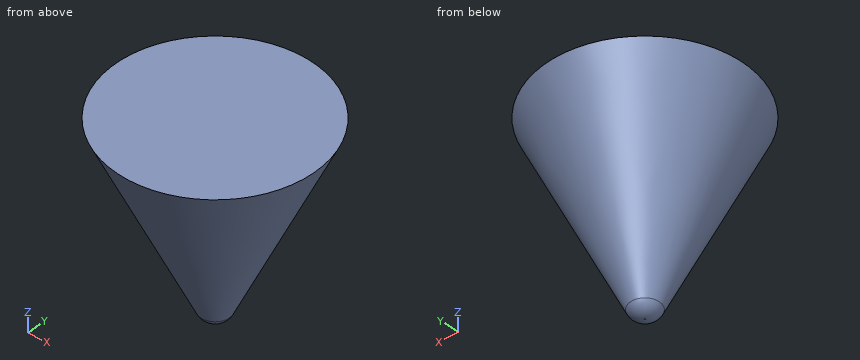
from build123d import *

# Parameters (mm, degrees)
F1_R     = 4.699
F2_DEPTH = 6.35
F2_TAPER = 25
F3_R     = 2.54
F4_R     = 4.699
F5_DEPTH = 25.4
F5_TAPER = -25


with BuildPart() as f2:
    # F1 (on offset) → F2 (new body)
    with BuildSketch(Plane.XY.offset(-25.4)):
        Circle(F1_R)
    extrude(amount=-F2_DEPTH, taper=F2_TAPER)

    # F3
    f3_edges = [f2.edges().sort_by_distance(p)[0] for p in [
        (-1.737946, 0, -31.75),
    ]]
    fillet(f3_edges, radius=F3_R)

    # F4 (on offset) → F5 (join)
    with BuildSketch(Plane.XY.offset(-25.4)):
        Circle(F4_R)
    extrude(amount=F5_DEPTH, taper=F5_TAPER)


solid = f2.part
The model under review builds one solid part; all positions refer to its coordinate system, in mm. Give positions to 0.01 mm unless a question says otherwise; leave off trailing zeros. Order: outer loops, then holes, each group sorted by start corner. A loop starts at its lowest first (then second) coordinate and runs counter-clockwise, first axis right, second up. Notation, with made-up numbers: M 39,-11.5 L 74,-11.5 A25 cw 74,23.5 Z; hole C 32.5,27 d6. An arc over 180 degrees is marked long. Use one line per item in the form item = value. Start each with the question number.
Item 1: We need section B-B on z = -21. Give the boundary of the cut face in (x, y), plus the area to 3 significant figures.
Item 2: Insertion check: pin 1 Ø6 at (y, z) = (-7, -12.5) entering from -X; pin 2 Ø4 at (x, z) = (4, -20.5) entering from +Y; pin 3 Ø1 at (x, y) = (-12, 12) entering from -Z. Each pin has a flat end and moves straight along its axis. Give the tip position at first contact, or say it passes through.
Item 3: We need section A-A on z = -26. Give the boundary of the cut face in (x, y), plus the area to 3 significant figures.
Item 4: To check wall thickness, follow line 1 along Y through (x, z) = (-4, -23.5); line 2 along Y through (x, z) = (-0.5, -30); line 3 along Z through (x, y) = (12.5, 0). State the ranges of each line that lie inside material, in increasing order. Write a range as from..to.
Completed:
q1.outline = C 0,0 d13.5
q1.area = 143 mm²
q2.pin_1 = -10.64
q2.pin_2 = 7.21
q2.pin_3 = -0.16
q3.outline = C 0,0 d8.84
q3.area = 61.4 mm²
q4.line_1 = -3.9..3.9
q4.line_2 = -2.5..2.5
q4.line_3 = -8.67..0
